Verification items for the finished model (mm, model axes). Face numbers are marked on the shaded views. Give positions to 0.01 mm unless a question says otherwise; leave off trailing zeros. Order: outer loops, then holes, each group sorted by start corner. A loop starts at its lowest first (then second) coordinate and runs counter-clockwise, first axis right, second up. Notation, with made-up numbers: (46, 81) - (64, 81) arc R17 ccw to (64, 105) - close; hole circle Ø10 at (-12.5, 87.25). An arc over 180 degrees is marked (long way). Answer as a JSON object with one key per item and string values.
```python
from build123d import *

# Parameters (mm, degrees)
CROQUIS1_R              = 1.25
SALIENTE_EXTRUIR1_DEPTH = 1.5
CORTAR_EXTRUIR1_DEPTH   = 0.5


with BuildPart() as part:
    # Croquis1 → Saliente-Extruir1 (new body)
    with BuildSketch(Plane(origin=(0, 0, 0), x_dir=(1, 0, 0), z_dir=(0, 1, 0))):
        Circle(CROQUIS1_R)
    extrude(amount=SALIENTE_EXTRUIR1_DEPTH)

    # Croquis2 one side → Revolución1 (revolve)
    with BuildSketch(Plane(origin=(0, 0, 0), x_dir=(0, 0, -1), z_dir=(1, 0, 0))):
        Polygon((0, 2.75), (0, 1.5), (1.25, 1.5), (2.5, 2.75), align=None)
    revolve(axis=Axis((0, 2.75, 0), (0, -1, 0)))

    # Croquis3 → Cortar-Extruir1 (cut)
    with BuildSketch(Plane(origin=(0, 2.75, 0), x_dir=(1, 0, 0), z_dir=(0, 1, 0))):
        Polygon((1.443375673, 0), (0.721687836, 1.25), (-0.721687836, 1.25), (-1.443375673, 0), (-0.721687836, -1.25), (0.721687836, -1.25), align=None)
    extrude(amount=-CORTAR_EXTRUIR1_DEPTH, mode=Mode.SUBTRACT)

    # Croquis4 one side → Revolución2 (revolve)
    with BuildSketch(Plane.XY):
        Polygon((0, 0), (0, -1), (1.25, 0), align=None)
    revolve(axis=Axis((0, 0, 0), (0, -1, 0)))


solid = part.part
```
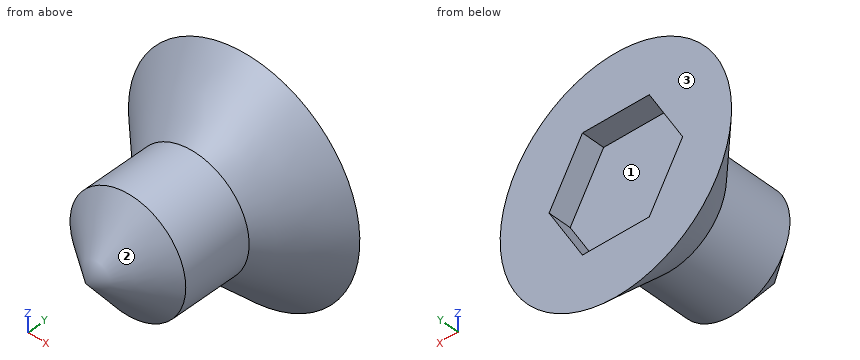
(1) Release check for a two-part mould opening along X. For the marked faces 1, 2 and 3 record: pulls with the +X half, pulls with the -X half, needs draft (parallel to the pull), parting line crosses it, or undercut.
Computed values:
{"face 1": "undercut", "face 2": "parting line crosses it", "face 3": "needs draft"}
(2) Gauge pin test, flat ends, axial feed: pin 1 Ø0.8 at (x, z) = (0, 0.5) entering from +Y; pin 2 Ø1 at (y, z) = (1, 1.5) entering from -X. Record the tip position at first contact, or that the pin passes through.
Computed values:
{"pin 1": "stops at y = 2.25", "pin 2": "stops at x = -0.75"}
(3) Section check B-B (y = 1.05). Record the cut outline in (x, z), then the cut area to 3 significant figures.
Computed values:
{"outline": "circle Ø2.5 at (0, 0)", "area": "4.91 mm²"}
(4) Material ranges on line 1 along X through (y, z) = (1.8, 0.5); line 2 along Y through (x, z) = (2.15, 0.9); line 3 along Y through (x, z) = (1.25, -1.65), recorded low to high. Write a range as [from, to].
Computed values:
{"line 1": "x = [-1.47, 1.47]", "line 2": "y = [2.58, 2.75]", "line 3": "y = [2.32, 2.75]"}
(5) Section check A-A (y = 2.15). Record the cut outline in (x, z), then the cut area to 3 significant figures.
Computed values:
{"outline": "circle Ø3.8 at (0, 0)", "area": "11.3 mm²"}
